Read the model definition and answer for the solid it produces. Units are mm, in the model's axes. Face numbers are marked on the shaded views. A direction names the side the tool comes from. Give positions to 0.01 mm unless a question says otherwise; leave off trailing zeros. Loops run counter-clockwise (first coordinate to the right, second up) from the corner with the lowest first, then second, coordinate; pieces in that order, holes last.
(1) Each of these flat-tipped pins is pushed along its axis until it touches: P1, Ø1, axis at x = -7.5, z = 1.5, coming from the -Y side (3 decimals); P2, Ø1.5, axis at y = 5.5, z = 2.5, coming from the +X side; P3, Ø2, axis at y = -10, z = 2, coming from the -X side. Where does it stop, or does it pass through?
(2) Which of the six approach directions +Z, -Z, +X, -X, +Y, -Y give full straight-line access (tool end or side, diameter ignored) to the marked faces 1, 2 and 3?
(3) Find section B-B, the plane z = 3.25. Write down the section's boundary in (x, y) (3 decimals).
(4) Find section A-A, the plane x = 0. Write down the section's boundary in (y, z) (3 decimals).
(5) Find section C-C, the plane y = 6.25. Write down the section's boundary in (x, z), then the cut area to 3 significant figures.
(6) Straight lines are drawn through the part: probe 1 along X at (y, z) = (2, 1.15) (3 decimals); probe 2 along Y at (x, z) = (0, 1.8) (3 decimals); probe 3 along X at (y, z) = (-9, 1). For each, find the intervals that lie inside material, in ascending order.
(7) Find section D-D, the plane x = -8. Write down the section's boundary in (y, z) (3 decimals), then the cut area to 3 significant figures.
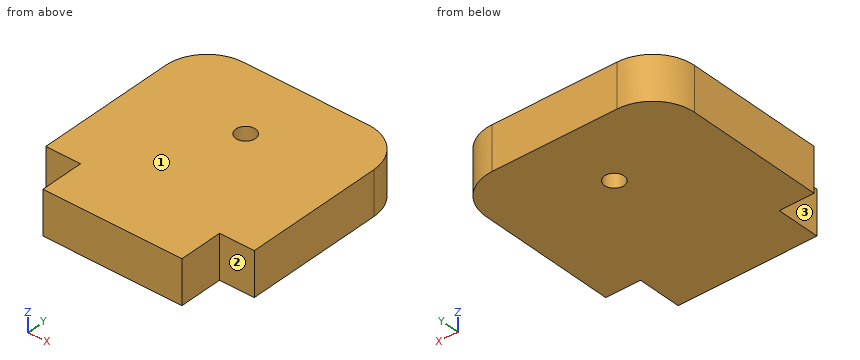
```python
from build123d import *

# Parameters (mm, degrees)
SKETCH2_R           = 0.889
BOSS_EXTRUDE1_DEPTH = 4


with BuildPart() as part:
    # Sketch2 → Boss-Extrude1 (new body)
    with BuildSketch(Plane.XY):
        with BuildLine():
            Line((-9.525, -8.255), (-6.35, -8.255))
            Line((-6.35, -8.255), (-6.35, -12.255))
            Line((-6.35, -12.255), (6.35, -12.255))
            Line((6.35, -12.255), (6.35, -8.255))
            Line((6.35, -8.255), (9.525, -8.255))
            Line((9.525, -8.255), (9.525, 4.445))
            ThreePointArc((9.525, 4.445), (8.409076836, 7.139076836), (5.715, 8.255))
            Line((5.715, 8.255), (-5.715, 8.255))
            ThreePointArc((-5.715, 8.255), (-8.409076836, 7.139076836), (-9.525, 4.445))
            Line((-9.525, 4.445), (-9.525, -8.255))
        make_face()
        with Locations((0, 1.905)):
            Circle(SKETCH2_R, mode=Mode.SUBTRACT)
    extrude(amount=BOSS_EXTRUDE1_DEPTH)


solid = part.part
```
Entries:
1. P1: stops at y = -8.255
1. P2: stops at x = 9.51
1. P3: stops at x = -6.35
2. face 1: +Z, +X, -X, +Y, -Y
2. face 2: +Z, -Z, +X, -Y
2. face 3: +Z, -Z, -X, -Y
3. outline: (-9.525, -8.255) - (-6.35, -8.255) - (-6.35, -12.255) - (6.35, -12.255) - (6.35, -8.255) - (9.525, -8.255) - (9.525, 4.445) arc R3.81 ccw to (5.715, 8.255) - (-5.715, 8.255) arc R3.81 ccw to (-9.525, 4.445) - close; hole circle Ø1.778 at (0, 1.905)
4. outline: (-12.255, 0) - (1.016, 0) - (1.016, 4) - (-12.255, 4) - close; (2.794, 0) - (8.255, 0) - (8.255, 4) - (2.794, 4) - close
5. outline: (-9.07, 0) - (9.07, 0) - (9.07, 4) - (-9.07, 4) - close
5. area: 72.6 mm2
6. probe 1: x = -9.525 to -0.884, 0.884 to 9.525
6. probe 2: y = -12.255 to 1.016, 2.794 to 8.255
6. probe 3: x = -6.35 to 6.35
7. outline: (-8.255, 0) - (7.494, 0) - (7.494, 4) - (-8.255, 4) - close
7. area: 63.0 mm2
